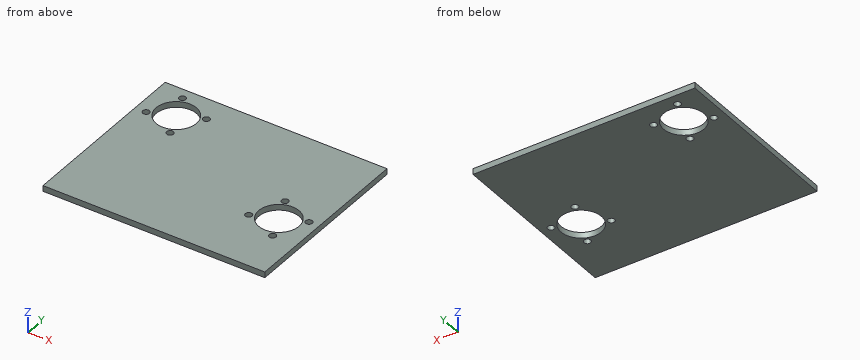
from build123d import *

# Parameters (mm, degrees)
SKETCH1_W           = 122
SKETCH1_H           = 99
SKETCH1_R           = 11.1125
SKETCH1_R_2         = 1.8542
BOSS_EXTRUDE1_DEPTH = 3.175


with BuildPart() as part:
    # Sketch1 → Boss-Extrude1 (new body)
    with BuildSketch(Plane.XY):
        with Locations((42, -30.5)):
            Rectangle(SKETCH1_W, SKETCH1_H)
        Circle(SKETCH1_R, mode=Mode.SUBTRACT)
        with Locations((-5.352449154, 12.936432586)):
            Circle(SKETCH1_R_2, mode=Mode.SUBTRACT)
        with Locations((-12.936432586, -5.352449154)):
            Circle(SKETCH1_R_2, mode=Mode.SUBTRACT)
        with Locations((12.936432586, 5.352449154)):
            Circle(SKETCH1_R_2, mode=Mode.SUBTRACT)
        with Locations((5.352449154, -12.936432586)):
            Circle(SKETCH1_R_2, mode=Mode.SUBTRACT)
        with Locations((84.431124445, -41.275)):
            Circle(SKETCH1_R, mode=Mode.SUBTRACT)
        with Locations((79.07867529, -28.338567414)):
            Circle(SKETCH1_R_2, mode=Mode.SUBTRACT)
        with Locations((71.494691859, -46.627449154)):
            Circle(SKETCH1_R_2, mode=Mode.SUBTRACT)
        with Locations((89.783573599, -54.211432586)):
            Circle(SKETCH1_R_2, mode=Mode.SUBTRACT)
        with Locations((97.367557031, -35.922550846)):
            Circle(SKETCH1_R_2, mode=Mode.SUBTRACT)
    extrude(amount=-BOSS_EXTRUDE1_DEPTH)


solid = part.part
Can you work these out from the model? Positions are in its coordinate system, mm. Coordinates: 2 decimals unless noted, no trailing zeros. Loops run counter-clockwise (first coordinate to the right, second up) from the corner with the lowest first, then second, coordinate; pieces in that order, holes last. Notation, with made-up numbers: M 52,43 L 105,43 A22 ccw 105,50 Z; hole C -6,39 d1. An arc over 180 degrees is marked long. Return JSON: item names as keys, results as strings. Group by question number.
Item 1: Imagine slicing it at B-B (x = 0). Please give me the cut outline in (y, z) (1 decimal).
Item 2: If I drill on L1, parallel to Y at x = 78.5, z = -0.35; L2, parallel to Y at x = 76, z = -1.3; L3, parallel to X at y = -5, z = -0.5, over which ranges is the centre line in solid material (lowest first)? Write a range as from..to.
Item 3: Imagine slicing it at A-A (y = 0). Please give me the cut outline in (x, z) (1 decimal), and give its area (3 significant figures).
Item 4: Imagine slicing it at C-C (z = -1.4). Give the number of separate pieces and of enclosed holes in the cut face, and give its area (3 significant figures).
Verdict:
{
 "1": {"outline": "M -80,-3.2 L -11.1,-3.2 L -11.1,0 L -80,0 Z; M 11.1,-3.2 L 19,-3.2 L 19,0 L 11.1,0 Z"},
 "2": {"L1": "y = -80..-50.67, -31.88..-30.1, -26.58..19", "L2": "y = -80..-48.51, -34.04..19", "L3": "x = -19..-14.76, -11.12..-9.92, 9.92..103"},
 "3": {"outline": "M -19,-3.2 L -11.1,-3.2 L -11.1,0 L -19,0 Z; M 11.1,-3.2 L 103,-3.2 L 103,0 L 11.1,0 Z", "area": "317 mm^2"},
 "4": {"separate pieces": "1", "enclosed holes": "10", "area": "11,200 mm^2"}
}
